Build history of the part. All positions in model axes, mm. Round coordinates to 2 decimals unless told otherwise and drop trailing zeros. Write each loop counter-clockwise with the first axis right and the second up, starting at its lowest first coordinate (ties: lowest second). Pieces come first, ordered by that corner, then holes. Notation, with made-up numbers: (86, 54.5) -> (114, 54.5) arc R25 cw to (114, 69.5) -> close; hole circle Ø5 at (34, 68). An arc over 180 degrees is marked (long way). Return JSON: item names as keys, results as strings.
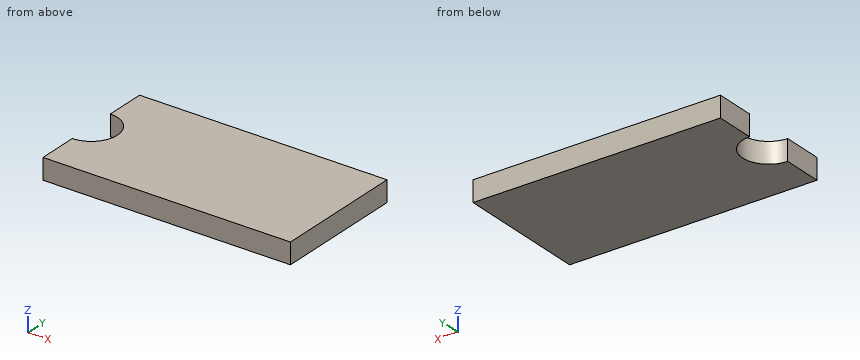
Autodesk Inventor part; units mm, degrees
ref_plane "YZ Plane" through (0, 0, 0) normal (1, 0, 0) x (0, 1, 0)
ref_plane "XZ Plane" through (0, 0, 0) normal (0, 1, 0) x (-1, 0, 0)
ref_plane "XY Plane" through (0, 0, 0) normal (0, 0, 1) x (1, 0, 0)
sketch "Sketch1" plane through (0, 0, 0) normal (0, 0, 1) x (1, 0, 0)
  line L0 (-11.85, -6.35) -> (11.85, -6.35)
  line L1 (11.85, -6.35) -> (11.85, 6.35)
  line L2 (11.85, 6.35) -> (-11.85, 6.35)
  line L3 (-11.85, 6.35) -> (-11.85, 2.5)
  line L4 (-11.85, -6.35) -> (11.85, 6.35) construction
  line L5 (11.85, -6.35) -> (-11.85, 6.35) construction
  arc A0 (-11.85, -2.5) -> (-11.85, 2.5) centre (-11.85, 0) ccw
  line L6 (-11.85, 2.5) -> (-11.85, -2.5) construction
  line L7 (-11.85, -2.5) -> (-11.85, -6.35)
  line L8 (-11.85, 0) -> (0, 0) construction
  dimension "d0" = 12.7
  dimension "d1" = 23.7
  dimension "d2" = 2.5
extrude "Extrusion1" add sketch "Sketch1" along normal blind 2
properties part number "LED Backing"
Q1. Saw through at B-B on y = 0. List the corners of the cut face in (x, z), then the cut area to 3 significant figures.
Verdict:
{"outline": "(-9.35, 0) -> (11.85, 0) -> (11.85, 2) -> (-9.35, 2) -> close", "area": "42.4 mm²"}
Q2. Wall check: L1, parallel to X at y = -0.25, z = 1.7; L2, parallel to X at y = 1, z = 1.45. Give the ranges that are in metal, low to high.
Verdict:
{"L1": "x = -9.36 to 11.85", "L2": "x = -9.56 to 11.85"}
Q3. Saw through at A-A on z = 1.4. List the corners of the cut face in (x, y).
Verdict:
{"outline": "(-11.85, -6.35) -> (11.85, -6.35) -> (11.85, 6.35) -> (-11.85, 6.35) -> (-11.85, 2.5) arc R2.5 cw to (-11.85, -2.5) -> close"}
